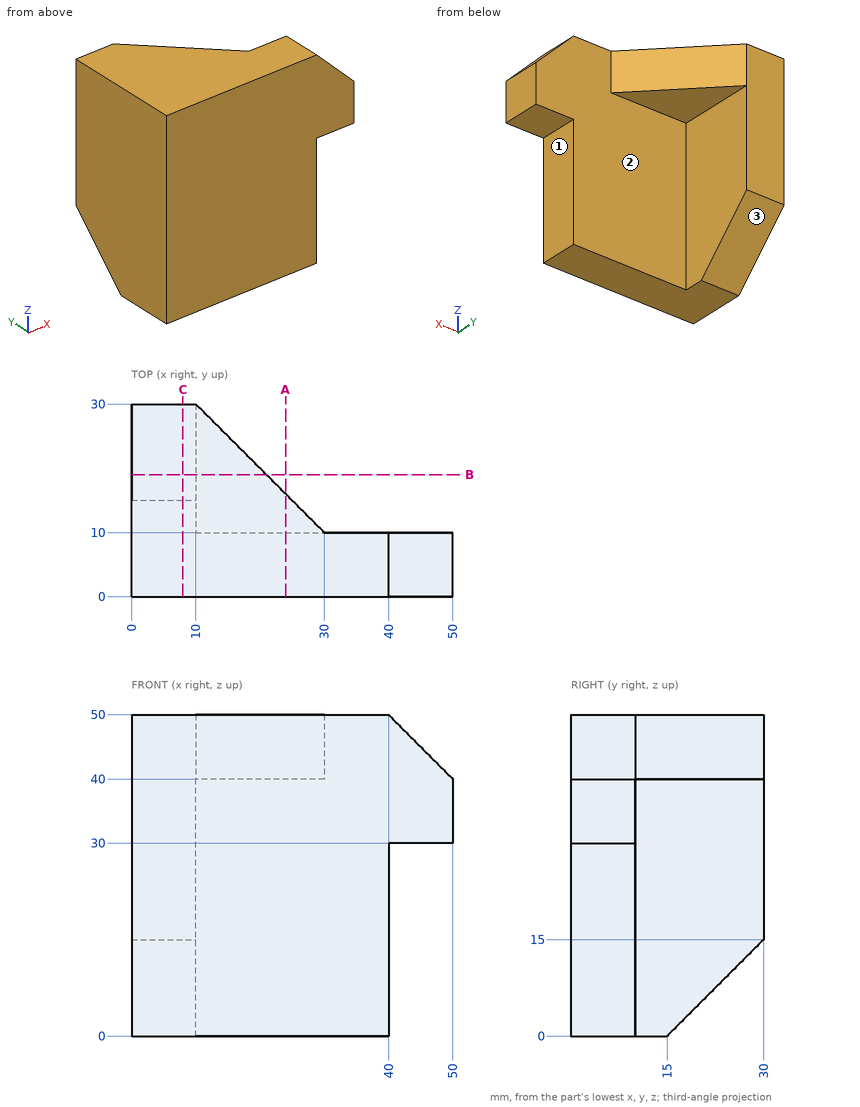
Geometry check sheet. Reference: drawing and pictorial views, mm from the part's lowest x, y, z. A direction names the side the tool comes from. Round coordinates to 2 decimals unless told otherwise and drop trailing zeros. Order: outer loops, then holes, each group sorted by start corner. A loop starts at its lowest first (then second) coordinate and runs counter-clockwise, first axis right, second up. Notation, with made-up numbers: M 71.5,46.5 L 120.5,46.5 A17 ccw 120.5,70.5 Z; hole C -39.75,-18 d4. An arc over 180 degrees is marked long. One line per item, written item: value. Start each with the question number.
1. Section check C-C on x = 8. Enter the section's corners in (y, z), and give its area (3 significant figures).
2. Scan lines: line 1 along X through (y, z) = (22, 26); line 2 along Z through (x, y) = (20, 17). Record each from-to range of solid material in increasing order.
3. Access from +Z, -Z, +X, -X, +Y, -Y to the whole of each face (thin tool, end or side, straight path). Record for the marked faces 1, 2 and 3.
4. Section check B-B on y = 19. Enter the section's corners in (x, z).
5. Gauge pin test, flat ends, axial feed: P1, Ø2, axis at x = 23.5, y = 11.5, coming from the -Z side; P2, Ø4, axis at x = 17.5, y = 24.5, coming from the +Z side; P3, Ø4, axis at x = 18.5, z = 35, coming from the +Y side; P4, Ø3, axis at x = 45.5, y = 6.5, coming from the -Z side. Record the tip position at first contact, or that the pin passes through.
6. Section check A-A on x = 24. Enter the section's corners in (y, z), and give its area (3 significant figures).
Results found:
1. outline: M 0,0 L 15,0 L 30,15 L 30,50 L 0,50 Z
1. area: 1,390 mm^2
2. line 1: 0 to 10
2. line 2: 40 to 50
3. face 1: -Z, +X, +Y, -Y
3. face 2: -Z, +X, +Y
3. face 3: -Z, +X, -X, +Y
4. outline: M 0,4 L 10,4 L 10,40 L 21,40 L 21,50 L 0,50 Z
5. P1: z = 40
5. P2: z = 50
5. P3: y = 10
5. P4: z = 30
6. outline: M 0,0 L 10,0 L 10,40 L 16,40 L 16,50 L 0,50 Z
6. area: 560 mm^2
